from build123d import *

# Parameters (mm, degrees)
BOX004_W                    = 3
BOX004_H                    = 31
BOX004_DEPTH                = 14
BOX003_W                    = 2
BOX003_H                    = 33
BOX003_DEPTH                = 11.2
BOX002_W                    = 3
BOX002_H                    = 35
BOX002_DEPTH                = 26
EXTRUDE_DEPTH               = 5
EXTRUDE001_DEPTH            = 5
THICKNESS_T                 = 1
BOX_W                       = 12
BOX_H                       = 31
BOX_DEPTH                   = 15
BOX001_W                    = 13
BOX001_H                    = 34
BOX001_DEPTH                = 14
CYLINDER001_W               = 48
CYLINDER001_H               = 15
CYLINDER001_ANGLE           = 60
CYLINDER001_PLACEMENT_ANGLE = 60
CYLINDER_W                  = 51
CYLINDER_H                  = 15
CYLINDER_ANGLE              = 60
CYLINDER_PLACEMENT_ANGLE    = 60


with BuildPart() as slot_wall_cutout2:
    # Box004 → Box004 (new body)
    with BuildSketch(Plane(origin=(-1, 7, 14), x_dir=(1, 0, 0), z_dir=(0, 0, 1))):
        with Locations((1.5, 15.5)):
            Rectangle(BOX004_W, BOX004_H)
    extrude(amount=BOX004_DEPTH)


with BuildPart() as slot_wall_cutout1:
    # Box003 → Box003 (new body)
    with BuildSketch(Plane(origin=(-0.5, 6, 15), x_dir=(1, 0, 0), z_dir=(0, 0, 1))):
        with Locations((1, 16.5)):
            Rectangle(BOX003_W, BOX003_H)
    extrude(amount=BOX003_DEPTH)


with BuildPart() as wall_slot_finished:
    # Box002 → Box002 (new body)
    with BuildSketch(Plane(origin=(-1, 5, 0), x_dir=(1, 0, 0), z_dir=(0, 0, 1))):
        with Locations((1.5, 17.5)):
            Rectangle(BOX002_W, BOX002_H)
    extrude(amount=BOX002_DEPTH)

    # Cut003: cut slot wall cutout1
    add(slot_wall_cutout1.part, mode=Mode.SUBTRACT)

    # Cut004: cut slot wall cutout2
    add(slot_wall_cutout2.part, mode=Mode.SUBTRACT)


with BuildPart() as extrude_body:
    with BuildSketch(Plane(origin=(8.5, 45, 6), x_dir=(1, 0, 0), z_dir=(0, 1, 0))):
        with BuildLine():
            Line((5, 4), (-5, 4))
            Line((-5, 4), (-5, -3.142136))
            ThreePointArc((-5, -3.142136), (-2.53653, -3.783978), (0, -4))
            ThreePointArc((0, -4), (2.53653, -3.783978), (5, -3.142136))
            Line((5, -3.142136), (5, 4))
        make_face()
    extrude(amount=EXTRUDE_DEPTH)


with BuildPart() as extrude001:
    with BuildSketch(Plane(origin=(8.5, 45, 6), x_dir=(1, 0, 0), z_dir=(0, 1, 0))):
        with BuildLine():
            Line((5, 4), (-5, 4))
            Line((-5, 4), (-5, -3.142136))
            ThreePointArc((-5, -3.142136), (-2.53653, -3.783978), (0, -4))
            ThreePointArc((0, -4), (2.53653, -3.783978), (5, -3.142136))
            Line((5, -3.142136), (5, 4))
        make_face()
    extrude(amount=EXTRUDE001_DEPTH)


with BuildPart() as bolt_bottle_side_opening:
    # Thickness base: copy of Extrude body
    add(extrude_body.part)

    # Thickness
    thickness_openings = [bolt_bottle_side_opening.faces().sort_by_distance(p)[0] for p in [
        (8.5, 50, 5.862901),
    ]]
    offset(amount=THICKNESS_T, openings=thickness_openings)

    # Fusion: union Extrude body, Extrude001
    add(extrude_body.part)
    add(extrude001.part)


with BuildPart() as bolt_bottle_side_opening_1:
    # Fusion placement: moved
    add(bolt_bottle_side_opening.part.moved(Location((0, -7, 1))))


with BuildPart() as pullbay:
    # Box → Box (new body)
    with BuildSketch(Plane(origin=(2.5, 7, 2), x_dir=(1, 0, 0), z_dir=(0, 0, 1))):
        with Locations((6, 15.5)):
            Rectangle(BOX_W, BOX_H)
    extrude(amount=BOX_DEPTH)


with BuildPart() as cut_bay_from_case:
    # Box001 → Box001 (new body)
    with BuildSketch(Plane(origin=(2, 6, 0), x_dir=(1, 0, 0), z_dir=(0, 0, 1))):
        with Locations((6.5, 17)):
            Rectangle(BOX001_W, BOX001_H)
    extrude(amount=BOX001_DEPTH)

    # Cut001: cut pullBay
    add(pullbay.part, mode=Mode.SUBTRACT)


with BuildPart() as bottle_wall001:
    # Cylinder001 → Cylinder001 (revolve)
    with BuildSketch(Plane.XZ):
        with Locations((24, 7.5)):
            Rectangle(CYLINDER001_W, CYLINDER001_H)
    revolve(axis=Axis((0, 0, 0), (0, 0, 1)), revolution_arc=CYLINDER001_ANGLE)


with BuildPart() as bottle_wall001_1:
    # Cylinder001 placement: moved
    add(bottle_wall001.part.moved(Location((8.5, -7, 0))).rotate(Axis((8.5, -7, 0), (0, 0, 1)), CYLINDER001_PLACEMENT_ANGLE))


with BuildPart() as fusion002:
    # Cylinder → Cylinder (revolve)
    with BuildSketch(Plane.XZ):
        with Locations((25.5, 7.5)):
            Rectangle(CYLINDER_W, CYLINDER_H)
    revolve(axis=Axis((0, 0, 0), (0, 0, 1)), revolution_arc=CYLINDER_ANGLE)


with BuildPart() as fusion002_1:
    # Cylinder placement: moved
    add(fusion002.part.moved(Location((8.5, -7, 0))).rotate(Axis((8.5, -7, 0), (0, 0, 1)), CYLINDER_PLACEMENT_ANGLE))

    # Cut: cut bottle_wall001
    add(bottle_wall001_1.part, mode=Mode.SUBTRACT)


with BuildPart() as fusion002_2:
    # Cut placement: moved
    add(fusion002_1.part.moved(Location((0, -2, 0))))

    # Fusion001: union cut bay from case
    add(cut_bay_from_case.part)

    # Cut002: cut bolt_bottle_side_opening
    add(bolt_bottle_side_opening_1.part, mode=Mode.SUBTRACT)

    # Fusion002: union wall slot finished
    add(wall_slot_finished.part)


solid = fusion002_2.part
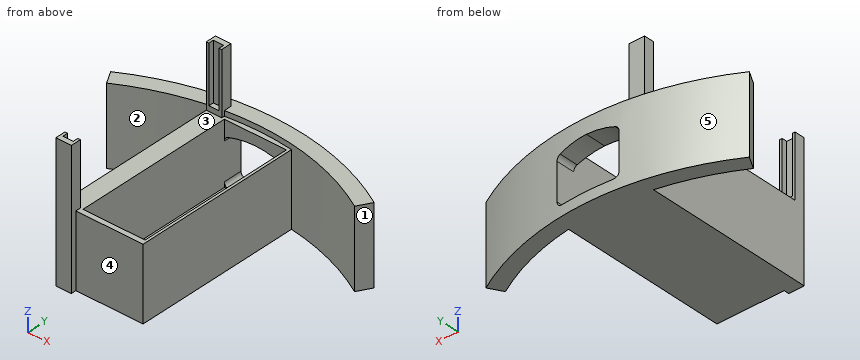
Geometry check sheet. Reference: the model listing, model coordinates, mm. Face numbers are marked on the shaded views. A direction names the side the tool comes from. Give positions to 0.01 mm unless a question says otherwise; leave off trailing zeros. Loops run counter-clockwise (first coordinate to the right, second up) from the corner with the lowest first, then second, coordinate; pieces in that order, holes last.
(1) Section check D-D on z = 5.25. Record the cut outline in (x, y), then the cut area to 3 significant figures.
From the geometry:
outline: (-17, 35.17) - (-15.5, 32.57) arc R48 cw to (-1, 38.05) - (-1, 5) - (2, 5) - (2, 6) - (15, 6) - (15, 38.56) arc R48 cw to (32.5, 32.57) - (34, 35.17) arc R51 ccw to (14.5, 41.65) - (14.5, 7) - (2.5, 7) - (2.5, 41.65) arc R51 ccw to start
area: 264 mm2
(2) Thickness scan on L1, parallel to X at y = 16.5, z = 9; L2, parallel to X at y = 38.5, z = 15.5; L3, parallel to Z at x = 13, y = 36. Record the ranges inside material, lowest first.
From the geometry:
L1: x = -1 to 2.5, 14.5 to 15
L2: x = -1 to -0.5, 1.5 to 2
L3: z = 0 to 2
(3) Set-up check for the marked faces 1 and 2: record each of +Z, -Z, +X, -X, +Y, -Y from which the full face is reachable in a straight line by a thin tool's end or side.
From the geometry:
face 1: +Z, -Z, +X, -Y
face 2: +Z, -Z, -Y
(4) Section check C-C on y = 22. Record the cut outline in (x, z).
From the geometry:
outline: (-1, 0) - (15, 0) - (15, 14) - (14.5, 14) - (14.5, 2) - (2.5, 2) - (2.5, 14) - (-1, 14) - close
(5) Section check B-B on x = 5.5. Record the cut outline in (y, z), then the cut area to 3 significant figures.
From the geometry:
outline: (6, 0) - (41.91, 0) - (41.91, 2) - (7, 2) - (7, 14) - (6, 14) - close; (38, 11.72) - (41.91, 11.72) - (41.91, 15) - (38.91, 15) - (38.91, 14) - (38, 14) - close
area: 95.8 mm2
(6) Section check A-A on z = 21.5. Record the cut outline in (x, y).
From the geometry:
outline: (-1, 5) - (2, 5) - (2, 7) - (1.5, 7) - (1.5, 6) - (-0.5, 6) - (-0.5, 7) - (-1, 7) - close; (-1, 38) - (-0.5, 38) - (-0.5, 39) - (1.5, 39) - (1.5, 38) - (2, 38) - (2, 40) - (-1, 40) - close
(7) Release check for a two-part mould opening along Y. For the marked faces 3, 4 and 5 record: released by +Y, released by -Y, zero draft, split by the parting line, or undercut.
From the geometry:
face 3: undercut
face 4: released by -Y
face 5: released by +Y
(8) Depth check by flat-ended pin: pin 1 Ø9.5 at (x, z) = (9.5, 5) entering from +Y; pin 2 Ø13 at (x, y) = (11.5, 29) entering from +Z; pin 3 Ø4 at (y, z) = (23.5, 10.5) entering from -X. Enter the tip coordinate at first touch or a pass-through.
From the geometry:
pin 1: stops at y = 42
pin 2: stops at z = 14
pin 3: stops at x = -1
